Autodesk Inventor part; units mm, degrees
ref_plane "YZ Plane" through (0, 0, 0) normal (1, 0, 0) x (0, 1, 0)
ref_plane "XZ Plane" through (0, 0, 0) normal (0, 1, 0) x (-1, 0, 0)
ref_plane "XY Plane" through (0, 0, 0) normal (0, 0, 1) x (1, 0, 0)
sketch "Szkic1" plane through (0, 0, 0) normal (0, 1, 0) x (-1, 0, 0)
  line L0 (-75, 75) -> (75, 75)
  line L1 (75, 75) -> (75, -75)
  line L2 (75, -75) -> (-75, -75)
  line L3 (-75, -75) -> (-75, 75)
  line L4 (-75, 75) -> (75, -75) construction
  line L5 (75, 75) -> (-75, -75) construction
  point P0 (0, 0)
  dimension "d0" = 150
  dimension "d1" = 150
extrude "Wyciągnięcie proste1" add sketch "Szkic1" along normal blind 70
sketch "Szkic2" plane through (0, 70, 0) normal (0, 1, 0) x (1, 0, 0)
  line L0 (-75, 75) -> (-75, -75)
  line L1 (75, 75) -> (-75, 75)
  line L2 (75, -75) -> (75, 75)
  line L3 (75, 75) -> (-75, 75)
  line L4 (-75, 75) -> (-75, -75)
  line L5 (-75, -75) -> (75, -75)
  line L6 (75, -75) -> (75, 75)
  circle A0 centre (0, 0) radius 75
  dimension "d4" = 150
extrude "Wyciągnięcie proste2" add sketch "Szkic2" along normal blind 350 contours A0
sketch "Szkic3" plane through (0, 420, 0) normal (0, 1, 0) x (1, 0, 0)
  circle A0 centre (0, 0) radius 75
  circle A1 centre (0, 0) radius 65
  line L0 (0, 0) -> (-19.4114, 72.4444)
  line L1 (0, 0) -> (19.4114, 72.4444)
  arc A2 (75, 0) -> (0, 75) centre (0, 0) ccw
  line L2 (0, 0) -> (0, 75)
  line L3 (75, 75) -> (-75, 75)
  point P0 (-16.8232, 62.7852)
  point P1 (16.8232, 62.7852)
  dimension "d7" = 130
  dimension "d8" = 15
  dimension "d9" = 15
extrude "Wyciągnięcie proste3" add sketch "Szkic3" along normal blind 150 contours L1 A1 L2 A0 | A0 L2 A1 L0
sketch "Szkic4" plane through (0, 570, 0) normal (0, 1, 0) x (1, 0, 0)
  circle A0 centre (0, 0) radius 75
  dimension "d12" = 150
extrude "Wyciągnięcie proste4" add sketch "Szkic4" along normal blind 20
sketch "Szkic5" plane through (0, 420, 0) normal (0, 1, 0) x (1, 0, 0)
  circle A0 centre (0, 0) radius 12.5
  dimension "d15" = 25
sketch "Szkic6" plane through (0, 570, 0) normal (0, -1, 0) x (1, 0, 0)
  circle A0 centre (0, 0) radius 12.5
  dimension "d18" = 25
hole "Otwór1" at (0, 420, 0) direction (0, -1, 0) diameter 25 depth 10
hole "Otwór2" at (0, 570, 0) direction (0, 1, 0) diameter 25 depth 10
equation "\"PromieńGięcia\" = Grubość"
equation "\"SzerokośćGięciaPodcięcia\" = Grubość"
equation "\"GłębokośćGięciaPodcięcia\" = 0.5 * Grubość"
equation "\"RozmiarPodcięciaNarożnika\" = 4 * Grubość"
equation "\"MinimalnaPozostałość\" = 2 * Grubość"
equation "\"PromieńPrzejścia\" = PromieńGięcia"
equation "\"Rozmiar_promienia_Jacobiego\" = PromieńGięcia"
equation "\"Wielk_odstępu\" = Grubość"
properties part number "1przegub"
Verification items for the finished model (mm, model axes). A direction names the side the tool comes from. Give positions to 0.01 mm unless a question says otherwise; leave off trailing zeros. Loops run counter-clockwise (first coordinate to the right, second up) from the corner with the lowest first, then second, coordinate; pieces in that order, holes last.
1. Section check A-A, the plane z = -47.5. Enter the section's corners in (x, y), then the cut area to 3 significant figures.
2. Set-up check for faces 4 (the flat face through (60, 70, 57)), 5 (the cylindrical face through (-3.755, 414.93, 11.923)), 6 (the flat face through (60, 70, -57)): record each of +Z, -Z, +X, -X, +Y, -Y from which the full face is reachable in a straight line by a thin tool's end or side.
3. Section check C-C, the plane x = 5.5. Enter the section's corners in (y, z), then the cut area to 3 significant figures.
4. Go/stop test with flat-tipped pins: pin 1 Ø12 at (x, y) = (52, 429.5) entering from +Z; pin 2 Ø6 at (y, z) = (126.5, 59.5) entering from -X; pin 3 Ø10 at (x, y) = (30, 118.5) entering from -Z; pin 4 Ø6 at (y, z) = (196.5, 11.5) entering from +X. Record where each tip stops, or that it passes through.
5. Section check D-D, the plane y = 369.5. Enter the section's corners in (x, z), then the cut area to 3 significant figures.
6. Thickness scan on line 1 (X direction, y = 415.75, z = 0); line 2 (Y direction, x = 12, z = 33.5). Record the ranges inside material, lowest first.
7. Mould release check, pull along Z, two halves, no side actions. Record for faces 1 (the cylindrical face through (-3.755, 575.07, -11.923)), 2 (the cylindrical face through (0, 494, -65)), 3 (the flat face through (-1, 570, 17)): released by +Z, released by -Z, zero draft, split by the parting line, or undercut.
8. Section check B-B, the plane x = 64. Enter the section's corners in (y, z), then the cut area to 3 significant figures.
Geometry says:
1. outline: (-75, 0) - (75, 0) - (75, 70) - (58.04, 70) - (58.04, 420) - (-58.04, 420) - (-58.04, 70) - (-75, 70) - close; (-58.04, 570) - (58.04, 570) - (58.04, 590) - (-58.04, 590) - close
1. area: 53,500 mm2
2. face 4: +Z, +X, +Y
2. face 5: none
2. face 6: -Z, +X, +Y
3. outline: (0, -75) - (70, -75) - (70, -74.8) - (590, -74.8) - (590, 74.8) - (570, 74.8) - (570, 11.22) - (580, 11.22) - (580, -11.22) - (570, -11.22) - (570, -64.77) - (420, -64.77) - (420, -11.22) - (410, -11.22) - (410, 11.22) - (420, 11.22) - (420, 74.8) - (70, 74.8) - (70, 75) - (0, 75) - close
3. area: 66,900 mm2
4. pin 1: passes through
4. pin 2: stops at x = -49.32
4. pin 3: stops at z = -70.71
4. pin 4: stops at x = 74.52
5. outline: circle Ø150 at (0, 0)
5. area: 17,700 mm2
6. line 1: x = -75 to -12.5, 12.5 to 75
6. line 2: y = 0 to 420, 570 to 590
7. face 1: undercut
7. face 2: released by +Z
7. face 3: zero draft
8. outline: (0, -75) - (70, -75) - (70, -39.1) - (420, -39.1) - (420, 39.1) - (70, 39.1) - (70, 75) - (0, 75) - close; (570, -39.1) - (590, -39.1) - (590, 39.1) - (570, 39.1) - close
8. area: 39,400 mm2
